from build123d import *

# Parameters (mm, degrees)
SKETCH1_R           = 37.5
BOSS_EXTRUDE1_DEPTH = 32.5
SKETCH2_OUTSIDE_W   = 603.232
SKETCH2_OUTSIDE_H   = 623.998
SKETCH2_OUTSIDE_R   = 67.116968793
CUT_EXTRUDE1_DEPTH  = 122.391669813
CUT_EXTRUDE1_DRAFT  = -60
SKETCH3_OUTSIDE_W   = 603.232
SKETCH3_OUTSIDE_H   = 623.998
SKETCH3_OUTSIDE_R   = 67.116968793
CUT_EXTRUDE2_DEPTH  = 122.391669813
CUT_EXTRUDE2_DRAFT  = -60
SKETCH4_R           = 50
SKETCH4_R_2         = 37.5
BOSS_EXTRUDE2_DEPTH = 50


with BuildPart() as part:
    # Sketch1 → Boss-Extrude1 (new, symmetric)
    with BuildSketch(Plane.XY):
        Polygon((0, 77.5), (-67.116968793, 38.75), (-67.116968793, -38.75), (0, -77.5), (67.116968793, -38.75), (67.116968793, 38.75), align=None)
        Circle(SKETCH1_R, mode=Mode.SUBTRACT)
    extrude(amount=BOSS_EXTRUDE1_DEPTH, both=True)


with BuildPart() as cut_extrude1_tool:
    # Sketch2 outside → Cut-Extrude1 (with draft: the straight prism first)
    with BuildSketch(Plane.XY.offset(32.5)):
        Rectangle(SKETCH2_OUTSIDE_W, SKETCH2_OUTSIDE_H)
        Circle(SKETCH2_OUTSIDE_R, mode=Mode.SUBTRACT)
    extrude(amount=-CUT_EXTRUDE1_DEPTH)
    # Cut-Extrude1: the draft: its side faces are tilted about the plane it starts from
    cut_extrude1_sides = [cut_extrude1_tool.faces().sort_by_distance(p)[0] for p in [
        (0, -311.999, -28.695834907),
        (301.616, 0, -28.695834907),
        (0, 311.999, -28.695834907),
        (-301.616, 0, -28.695834907),
        (-67.116968793, 0, -28.695834907),
    ]]
    draft(cut_extrude1_sides, Plane.XY.offset(32.5), CUT_EXTRUDE1_DRAFT)


with BuildPart() as part_1:
    add(part.part)

    # Cut-Extrude1: cut by cut_extrude1_tool
    add(cut_extrude1_tool.part, mode=Mode.SUBTRACT)


with BuildPart() as cut_extrude2_tool:
    # Sketch3 outside → Cut-Extrude2 (with draft: the straight prism first)
    with BuildSketch(Plane(origin=(0, 0, -32.5), x_dir=(-1, 0, 0), z_dir=(0, 0, -1))):
        Rectangle(SKETCH3_OUTSIDE_W, SKETCH3_OUTSIDE_H)
        Circle(SKETCH3_OUTSIDE_R, mode=Mode.SUBTRACT)
    extrude(amount=-CUT_EXTRUDE2_DEPTH)
    # Cut-Extrude2: the draft: its side faces are tilted about the plane it starts from
    cut_extrude2_sides = [cut_extrude2_tool.faces().sort_by_distance(p)[0] for p in [
        (0, -311.999, 28.695834907),
        (-301.616, 0, 28.695834907),
        (0, 311.999, 28.695834907),
        (301.616, 0, 28.695834907),
        (67.116968793, 0, 28.695834907),
    ]]
    draft(cut_extrude2_sides, Plane(origin=(0, 0, -32.5), x_dir=(-1, 0, 0), z_dir=(0, 0, -1)), CUT_EXTRUDE2_DRAFT)


with BuildPart() as part_2:
    add(part_1.part)

    # Cut-Extrude2: cut by cut_extrude2_tool
    add(cut_extrude2_tool.part, mode=Mode.SUBTRACT)

    # Sketch4 → Boss-Extrude2 (add)
    with BuildSketch(Plane.XY.offset(32.5)):
        Circle(SKETCH4_R)
        Circle(SKETCH4_R_2, mode=Mode.SUBTRACT)
    extrude(amount=BOSS_EXTRUDE2_DEPTH)


solid = part_2.part
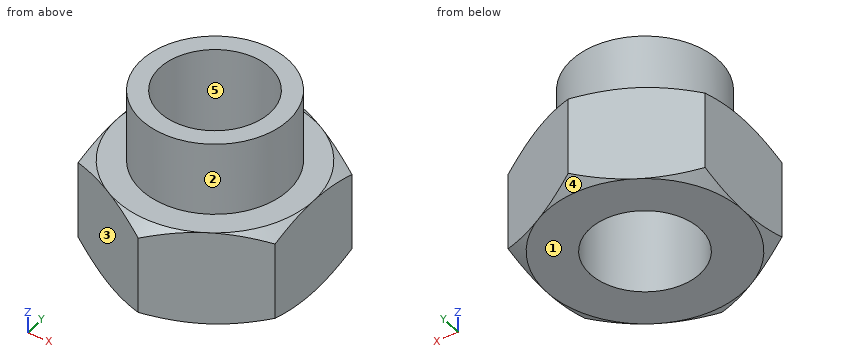
The listing builds one solid part. Answer for the finished solid, in the listing's coordinates (mm). Face numbers are marked on the shaded views. A direction names the side the tool comes from. Round coordinates to 2 decimals unless told otherwise and drop trailing zeros. Write each loop counter-clockwise with the first axis right and the second up, starting at its lowest first coordinate (ties: lowest second). Pieces come first, ordered by that corner, then holes. Notation, with made-up numbers: M -38,80.25 L 10,80.25 A10 cw 10,92.25 Z; hole C -19,50 d1. An arc over 180 degrees is marked long. Write each question's results on one line, items separated by ' | '. Start each with the question number.
Item 1: Straight lines are drawn through the part: probe 1 along Y at (x, z) = (0, 50); probe 2 along Z at (x, y) = (-48, 20.5); probe 3 along Y at (x, z) = (-1, -20). For each, find the intervals that lie inside material, in ascending order.
Item 2: Find section A-A on z = 11. Write down the section's boundary in (x, y), and give its area (3 significant figures).
Item 3: Given pin 1 Ø4 at (y, z) = (-21.5, 35.5) entering from +X; pin 2 Ø6 at (x, z) = (-26, 31.5) entering from -Y; pin 3 Ø2 at (y, z) = (-24, 65) entering from -X, each flat-ended and moving along its own axis, determine where each tip first touches the part or whether it passes through.
Item 4: Which of the six approach directions +Z, -Z, +X, -X, +Y, -Y give full straight-line access (tool end or side, diameter ignored) to the marked faces 1 and 2?
Item 5: Find section B-B on z = 59.5. Write down the section's boundary in (x, y).
Item 6: The mould has two halves that part along X. Classify the marked faces 3, 4 and 5: +X half, -X half, draft (parallel to the pull), parting line (faces both ways), or undercut.
Answer block:
1) probe 1: y = -50 to -37.5, 37.5 to 50 | probe 2: z = -32.5 to 32.5 | probe 3: y = -76.92 to -37.49, 37.49 to 76.92
2) outline: M -67.12,-38.75 L 0,-77.5 L 67.12,-38.75 L 67.12,38.75 L 0,77.5 L -67.12,38.75 Z; hole C 0,0 d75 | area: 11,200 mm²
3) pin 1: stops at x = 46.04 | pin 2: stops at y = -64.22 | pin 3: stops at x = -44.4
4) face 1: -Z, +X, -X, +Y, -Y | face 2: +Z
5) outline: C 0,0 d100; hole C 0,0 d75
6) face 3: -X half | face 4: parting line | face 5: undercut
